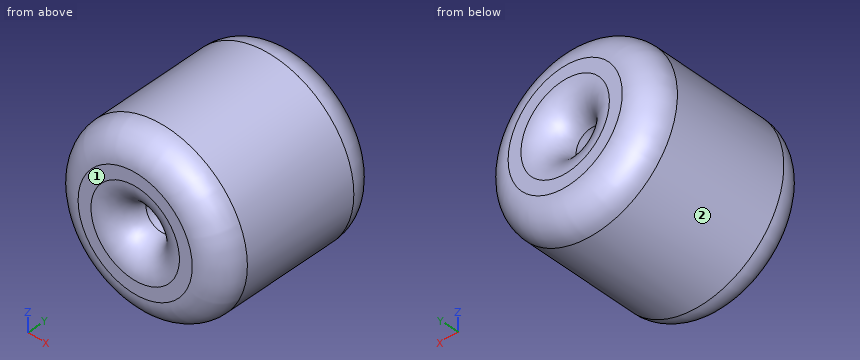
```python
from build123d import *

# Parameters (mm, degrees)
F0_R     = 60
F1_DEPTH = 120
F3_D     = 22
F4_R     = 20


with BuildPart() as f1:
    # F0 (on Front) → F1 (new body)
    with BuildSketch(Plane.XZ):
        Circle(F0_R)
    extrude(amount=F1_DEPTH)

    # F3 (through all)
    with Locations(Plane.XZ.offset(120)):
        with Locations((0, 0)):
            Hole(F3_D / 2)

    # F4
    f4_edges = [f1.edges().sort_by_distance(p)[0] for p in [
        (60, -60, 0),
        (-60, 0, 0),
        (-60, -120, 0),
        (-11, 0, 0),
        (-11, -120, 0),
    ]]
    fillet(f4_edges, radius=F4_R)


solid = f1.part
```
Input: part model. Units: mm. Frame: model coordinates. Face numbers are marked on the shaded views. Give positions to 0.01 mm unless a question says otherwise; leave off trailing zeros. Order: outer loops, then holes, each group sorted by start corner. A loop starts at its lowest first (then second) coordinate and runs counter-clockwise, first axis right, second up. Notation, with made-up numbers: (44.5, -29.5) -> (61.5, -29.5) arc R12 ccw to (61.5, -25.5) -> close; hole circle Ø10 at (-39.5, -25). An arc over 180 degrees is marked (long way). Write each question's results on one line, items separated by ' | '. Start each with the question number.
Item 1: Cut plane D-D on y = -8.5. Return the cut outline in (x, z), then the cut area to 3 significant figures.
Item 2: Cut plane C-C on y = -80.5. Return the cut outline in (x, z).
Item 3: Mould query, pull axis X, two halves, no side actions, for the marked faces 1 and 2. Classes: pulls with the +X half, pulls with the -X half, needs draft (parallel to the pull), parting line crosses it, or undercut.
Item 4: Cut plane B-B on z = 0. Return the cut outline in (x, y).
Item 5: Contact query for flat-ended pins moving along their axis: P1, Ø1.5, axis at x = 19, z = 9, coming from the -Y side; P2, Ø10, axis at y = -53.5, z = -7, coming from the +X side; P3, Ø17.5, axis at x = 0, z = 0, coming from the +Y side; P4, Ø4, axis at x = -47.5, z = -25, coming from the -Y side. Output: stop coordinate, or through.
Item 6: Line query: line 1 (Z direction, x = 0, y = -64); line 2 (Z direction, x = -12.5, y = -111); line 3 (X direction, y = -64, z = -4.5). Output: solid intervals per line, ascending.
Item 7: Cut plane A-A on x = 0. Return the cut outline in (y, z), then the cut area to 3 significant figures.
Established:
1) outline: circle Ø112.73 at (0, 0); hole circle Ø29.27 at (0, 0) | area: 9,310 mm^2
2) outline: circle Ø120 at (0, 0); hole circle Ø22 at (0, 0)
3) face 1: needs draft | face 2: parting line crosses it
4) outline: (-60, -100) arc R20 ccw to (-40, -120) -> (-31, -120) arc R20 ccw to (-11, -100) -> (-11, -20) arc R20 ccw to (-31, 0) -> (-40, 0) arc R20 ccw to (-60, -20) -> close; (11, -100) arc R20 ccw to (31, -120) -> (40, -120) arc R20 ccw to (60, -100) -> (60, -20) arc R20 ccw to (40, 0) -> (31, 0) arc R20 ccw to (11, -20) -> close
5) P1: y = -117.74 | P2: x = 59.97 | P3: through | P4: y = -116.24
6) line 1: -60 to -11, 11 to 60 | line 2: -55.31 to -6.94, 6.94 to 55.31 | line 3: -59.83 to -10.04, 10.04 to 59.83
7) outline: (-120, -40) arc R20 ccw to (-100, -60) -> (-20, -60) arc R20 ccw to (0, -40) -> (0, -31) arc R20 ccw to (-20, -11) -> (-100, -11) arc R20 ccw to (-120, -31) -> close; (-120, 31) arc R20 ccw to (-100, 11) -> (-20, 11) arc R20 ccw to (0, 31) -> (0, 40) arc R20 ccw to (-20, 60) -> (-100, 60) arc R20 ccw to (-120, 40) -> close | area: 11,100 mm^2
